Geometry check sheet. Reference: drawing and pictorial views, mm from the part's lowest x, y, z. A direction names the side the tool comes from. Give positions to 0.01 mm unless a question says otherwise; leave off trailing zeros. Write each loop counter-clockwise with the first axis right and the second up, starting at its lowest first coordinate (ties: lowest second). Pieces come first, ordered by that corner, then holes. Notation, with made-up numbers: (-22, 44) -> (18, 44) arc R16 cw to (18, 70) -> close; hole circle Ø9 at (-35, -2). An arc over 180 degrees is marked (long way). Return JSON: item names as keys, results as strings.
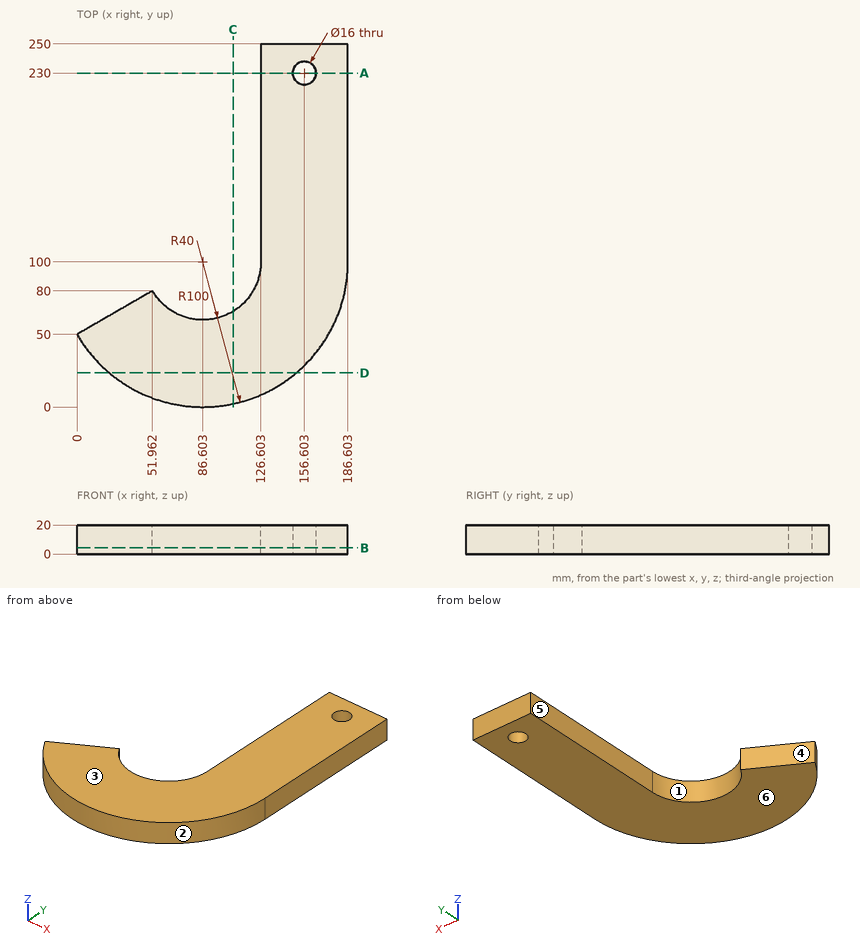
(1) Cross-section at C-C on x = 107.5. Enter the section's corners in (y, z), then the cut area to 3 significant figures.
Reply:
{"outline": "(2.21, 0) -> (65.89, 0) -> (65.89, 20) -> (2.21, 20) -> close", "area": "1,270 mm^2"}
(2) Set-up check for the marked faces 5 and 6: record each of +Z, -Z, +X, -X, +Y, -Y from which the full face is reachable in a straight line by a thin tool's end or side.
Reply:
{"face 5": "+Z, -Z, -X, +Y", "face 6": "-Z, +X, -X, +Y, -Y"}
(3) Depth check by flat-ended pin: pin 1 Ø6 at (x, z) = (26, 3.5) entering from +Y. Enter the tip coordinate at first touch or a pass-through.
Reply:
{"pin 1": "y = 66.74"}
(4) Release check for a two-part mould opening along X. For the marked faces 1, 2, 3 and 4 record: pulls with the +X half, pulls with the -X half, needs draft (parallel to the pull), parting line crosses it, or undercut.
Reply:
{"face 1": "undercut", "face 2": "parting line crosses it", "face 3": "needs draft", "face 4": "pulls with the -X half"}
(5) Cross-section at B-B on z = 4.25. Enter the section's corners in (x, y).
Reply:
{"outline": "(0, 50) arc R100 ccw to (186.6, 100) -> (186.6, 250) -> (126.6, 250) -> (126.6, 100) arc R40 cw to (51.96, 80) -> close; hole circle Ø16 at (156.6, 230)"}
(6) Cross-section at D-D on y = 23.5. Enter the section's corners in (x, z) (1 decimal).
Reply:
{"outline": "(22.2, 0) -> (151, 0) -> (151, 20) -> (22.2, 20) -> close"}
(7) Thickness scan on L1, parallel to X at y = 230, z = 12; L2, parallel to X at y = 177, z = 5.75; L3, parallel to Y at x = 161, z = 14 (1 decimal). Record the ranges inside material, lowest first.
Reply:
{"L1": "126.6 to 148.6, 164.6 to 186.6", "L2": "126.6 to 186.6", "L3": "33.2 to 223.3, 236.7 to 250"}
(8) Cross-section at A-A on y = 230. Enter the section's corners in (x, z).
Reply:
{"outline": "(126.6, 0) -> (148.6, 0) -> (148.6, 20) -> (126.6, 20) -> close; (164.6, 0) -> (186.6, 0) -> (186.6, 20) -> (164.6, 20) -> close"}
